Verification items for the finished model (mm, model axes). A direction names the side the tool comes from. Coordinates: 2 decimals unless noted, no trailing zeros. Loops run counter-clockwise (first coordinate to the right, second up) from the corner with the lowest first, then second, coordinate; pieces in that order, holes last. Notation, with made-up numbers: (51, 33) - (56, 33) arc R33 ccw to (56, 66) - close; hole circle Ø8 at (12, 5.25). An arc over 180 degrees is marked (long way). One line per item, written item: value. Start each with the question number.
(1) Thickness scan on probe 1 along Y at (x, z) = (3.5, -3.75); probe 2 along Y at (x, z) = (-15.35, 0); probe 3 along Y at (x, z) = (-18.5, -0.5). Record the ranges inside material, lowest first. Write a range as [from, to].
(2) Section check A-A (x = -18.5). Record the boundary of the cut face in (y, z), plus the area to 3 significant figures.
(3) Section check B-B (x = 1). Record the boundary of the cut face in (y, z), plus the area to 4 significant figures.
(4) Section check C-C (z = 0). Count the separate pieces of the cut face and the enclosed holes in it, plus the area to 3 significant figures.
(5) Gauge pin test, flat ends, axial feed: P1, Ø6, axis at x = -6, y = 7.5, coming from the +Z side; P2, Ø5, axis at y = 1.5, z = -3, coming from the +X side. Record the tip position at first contact, or that the pin passes through.
(6) Set-up check for faces 1 (the face through (0, 11, 0)), 2 (the face through (-15, 0, 8.5)): record each of +Z, -Z, +X, -X, +Y, -Y from which the full face is reachable in a straight line by a thin tool's end or side.
(7) Draft check along X on faces 3 (the face through (-19.782, -3.955, 5.158)), 4 (the face through (0, -11, 0)), 5 (the face through (-17.5, 1.54, 4.42)), 6 (the face through (22.5, -0.2, 7.2)). Enter one of: +X half, -X half, draft (parallel to the pull), parting line (faces both ways), or undercut.
```python
from build123d import *

# Parameters (mm, degrees)
SKETCH_1_W          = 45
SKETCH_1_H          = 30
EXTRUDE_1_DEPTH     = 8.5
SKETCH_2_R          = 6.5
CUT_EXTRUDE_1_DEPTH = 5
SKETCH_3_R          = 4
CUT_EXTRUDE_2_DEPTH = 53
CHAMFER_1_SIZE      = 0.5
HOLE_WIZARD_M4_1_D  = 3.3
SKETCH_7_W          = 29
SKETCH_7_H          = 22
CUT_EXTRUDE_3_DEPTH = 53
FILLET_1_R          = 2
CHAMFER_2_SIZE      = 0.5


with BuildPart() as part:
    # 草图1 → 凸台-拉伸1 (new, symmetric)
    with BuildSketch(Plane.XY):
        Rectangle(SKETCH_1_W, SKETCH_1_H)
    extrude(amount=EXTRUDE_1_DEPTH, both=True)

    # 草图2 → 切除-拉伸1 (cut)
    with BuildSketch(Plane(origin=(22.5, 0, 0), x_dir=(0, 0, -1), z_dir=(1, 0, 0))):
        Circle(SKETCH_2_R)
    cut_extrude_1 = extrude(amount=-CUT_EXTRUDE_1_DEPTH, mode=Mode.SUBTRACT)

    # 镜向1: 切除-拉伸1 across plane
    add(cut_extrude_1.mirror(Plane(origin=(0, 0, 0), x_dir=(0, 0, 1), z_dir=(1, 0, 0))), mode=Mode.SUBTRACT)

    # 草图3 → 切除-拉伸2 (cut)
    with BuildSketch(Plane(origin=(17.5, 0, 0), x_dir=(0, 0, -1), z_dir=(1, 0, 0))):
        Circle(SKETCH_3_R)
    extrude(amount=-CUT_EXTRUDE_2_DEPTH, mode=Mode.SUBTRACT)

    # 倒角1
    chamfer_1_edges = [part.edges().sort_by_distance(p)[0] for p in [
        (22.5, 0, 6.5),
        (-22.5, 0, 6.5),
        (-17.5, 0, 4),
        (17.5, 0, 4),
    ]]
    chamfer(chamfer_1_edges, length=CHAMFER_1_SIZE)

    # M4 螺纹孔1 (through all)
    with Locations(Plane(origin=(0, 0, -8.5), x_dir=(-1, 0, 0), z_dir=(0, 0, -1))):
        with Locations((-18.5, 11), (18.5, 11), (-18.5, -11), (18.5, -11)):
            Hole(HOLE_WIZARD_M4_1_D / 2)

    # 草图7 → 切除-拉伸3 (cut)
    with BuildSketch(Plane(origin=(0, 0, -8.5), x_dir=(-1, 0, 0), z_dir=(0, 0, -1))):
        Rectangle(SKETCH_7_W, SKETCH_7_H)
    extrude(amount=-CUT_EXTRUDE_3_DEPTH, mode=Mode.SUBTRACT)

    # 圆角1
    fillet_1_edges = [part.edges().sort_by_distance(p)[0] for p in [
        (-14.5, -11, 0),
        (14.5, 11, 0),
        (-14.5, 11, 0),
        (14.5, -11, 0),
    ]]
    fillet(fillet_1_edges, radius=FILLET_1_R)

    # 倒角2
    chamfer_2_edges = [part.edges().sort_by_distance(p)[0] for p in [
        (-22.5, 0, 8.5),
        (0, -15, 8.5),
        (22.5, 0, 8.5),
        (0, -15, -8.5),
        (-22.5, 0, -8.5),
        (0, 15, -8.5),
        (22.5, 0, -8.5),
        (22.5, -15, 0),
        (-22.5, -15, 0),
        (-22.5, 15, 0),
        (22.5, 15, 0),
        (0, 15, 8.5),
    ]]
    chamfer(chamfer_2_edges, length=CHAMFER_2_SIZE)


solid = part.part
```
Responses:
1. probe 1: y = [-15, -11], [11, 15]
1. probe 2: y = [-15, -4], [4, 15]
1. probe 3: y = [-15, -12.65], [-9.35, -6.48], [6.48, 9.35], [12.65, 15]
2. outline: (-15, -8) - (-14.5, -8.5) - (-12.65, -8.5) - (-12.65, 8.5) - (-14.5, 8.5) - (-15, 8) - close; (-9.35, -8.5) - (9.35, -8.5) - (9.35, 8.5) - (-9.35, 8.5) - close; (12.65, -8.5) - (14.5, -8.5) - (15, -8) - (15, 8) - (14.5, 8.5) - (12.65, 8.5) - close; hole circle Ø13 at (0, 0)
2. area: 265 mm²
3. outline: (-15, -8) - (-14.5, -8.5) - (-11, -8.5) - (-11, 8.5) - (-14.5, 8.5) - (-15, 8) - close; (11, -8.5) - (14.5, -8.5) - (15, -8) - (15, 8) - (14.5, 8.5) - (11, 8.5) - close
3. area: 135.5 mm²
4. separate pieces: 2
4. enclosed holes: 4
4. area: 502 mm²
5. P1: passes through
5. P2: stops at x = 17.5
6. face 1: +Z, -Z
6. face 2: +Z, +X, -X, +Y, -Y
7. face 3: draft
7. face 4: undercut
7. face 5: -X half
7. face 6: +X half
